Job drawing, mm, ordinate dimensions from the low corner. One solid piece. Round coordinates to 2 decimals unless told otherwise and drop trailing zeros. Write each loop counter-clockwise with the first axis right and the second up, starting at its lowest first coordinate (ties: lowest second). Pieces come first, ordered by that corner, then holes. Notation, with made-up numbers: (3, 46.25) - (15, 46.25) arc R27 cw to (15, 65.25) - close; hole circle Ø11 at (-4, 65). An arc over 180 degrees is marked (long way). Write each question's results on one line, items separated by ' | '.
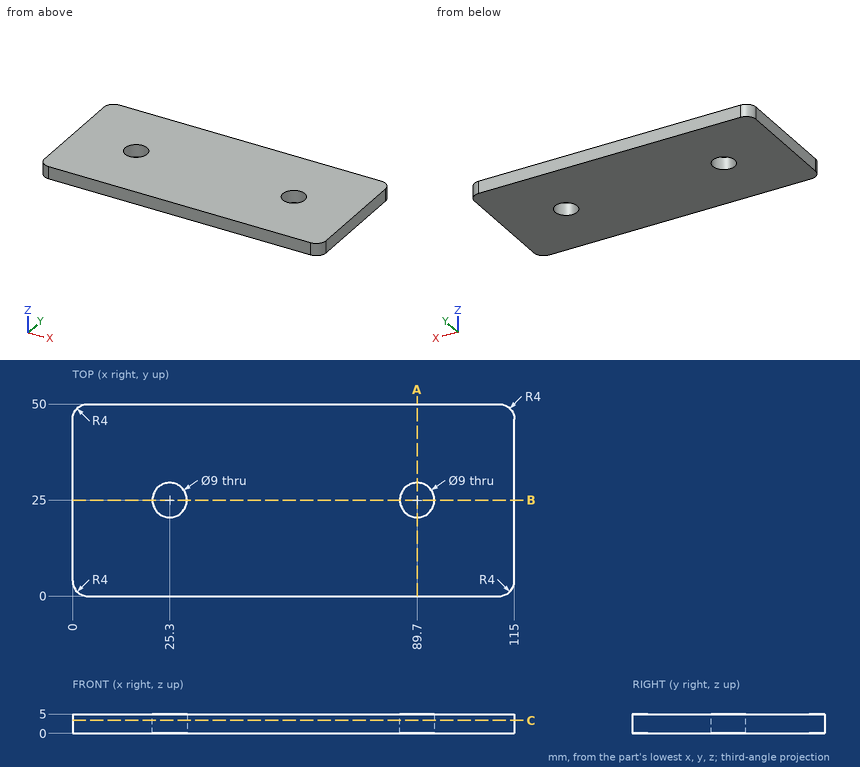
(1) Drill centre lines: probe 1 along Y at (x, z) = (89.7, 3.05); probe 2 along X at (y, z) = (24.5, 4.7); probe 3 along Y at (x, z) = (24, 0.5). Where is each one in solid material? Low to high. Write a range as [from, to].
Worked answers:
probe 1: y = [0, 20.5], [29.5, 50] | probe 2: x = [0, 20.83], [29.77, 85.23], [94.17, 115] | probe 3: y = [0, 20.69], [29.31, 50]
(2) Slice it at A-A, the plane x = 89.7. Write the cut outline in (y, z).
Worked answers:
outline: (0, 0) - (20.5, 0) - (20.5, 5) - (0, 5) - close; (29.5, 0) - (50, 0) - (50, 5) - (29.5, 5) - close
(3) Slice it at C-C, the plane z = 3.35. Write the cut outline in (x, y).
Worked answers:
outline: (0, 4) arc R4 ccw to (4, 0) - (111, 0) arc R4 ccw to (115, 4) - (115, 46) arc R4 ccw to (111, 50) - (4, 50) arc R4 ccw to (0, 46) - close; hole circle Ø9 at (25.3, 25); hole circle Ø9 at (89.7, 25)
(4) Flat gauge pin, fed straight in: pin 1 Ø5.5 at (x, y) = (25.3, 25) entering from -Z. Where does the tip first touch, or does it go through?
Worked answers:
pin 1: passes through
(5) Slice it at B-B, the plane y = 25. Write the cut outline in (x, z), and give its area (3 significant figures).
Worked answers:
outline: (0, 0) - (20.8, 0) - (20.8, 5) - (0, 5) - close; (29.8, 0) - (85.2, 0) - (85.2, 5) - (29.8, 5) - close; (94.2, 0) - (115, 0) - (115, 5) - (94.2, 5) - close | area: 485 mm2
